Design review of the part built by this model. Coordinates are the model's own, in mm. Face numbers are marked on the shaded views. A direction names the side the tool comes from. Coordinates: 2 decimals unless noted, no trailing zeros. Write each loop counter-clockwise with the first axis right and the second up, starting at its lowest first coordinate (ties: lowest second). Pieces come first, ordered by that corner, then holes. Notation, with made-up numbers: (16, 42) -> (34, 42) arc R21 ccw to (34, 80) -> close; hole circle Ø6 at (62, 50.5). An arc over 180 degrees is marked (long way). Write item = value, one per line. Start each with the question number.
```python
from build123d import *


with BuildPart() as part:
    # Sketch1 → Revolve1 (revolve)
    with BuildSketch(Plane(origin=(0, 0, 0), x_dir=(1, 0, 0), z_dir=(0, 1, 0)), mode=Mode.PRIVATE) as revolve1_sk:
        with BuildLine():
            Line((-7.95, 11.1), (-0.95, 11.1))
            Line((-0.95, 11.1), (-0.95, 6.1))
            Line((-0.95, 6.1), (0.95, 6.1))
            Line((0.95, 6.1), (0.95, 11.1))
            Line((0.95, 11.1), (7.95, 11.1))
            Line((7.95, 11.1), (7.95, 21))
            Line((7.95, 21), (6.75, 21))
            Line((6.75, 21), (3.703703704, 17.641044973))
            ThreePointArc((3.703703704, 17.641044973), (0, 16), (-3.703703704, 17.641044973))
            Line((-3.703703704, 17.641044973), (-6.75, 21))
            Line((-6.75, 21), (-7.95, 21))
            Line((-7.95, 21), (-7.95, 11.1))
        make_face()
    revolve(revolve1_sk.sketch.rotate(Axis((-3.715814159, 0, 0), (1, 0, 0)), 180), axis=Axis((-3.715814159, 0, 0), (1, 0, 0)))


solid = part.part
```
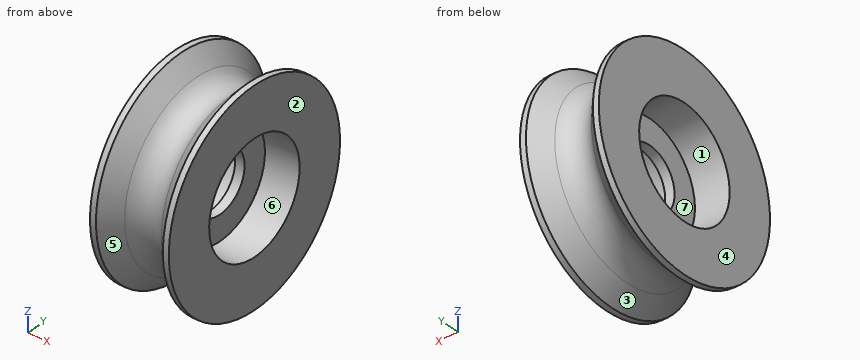
(1) Take a section at A-A, the plane y = 0. State the section outline as (x, z) points.
(2) For pin 1 Ø18 at (y, z) = (0, 0) entering from +X; pin 2 Ø3 at (x, y) = (-3, -15.5) entering from -Z; pin 3 Ø3 at (x, y) = (5.5, 5.5) entering from -Z, all flat-tipped, find the tip position at first contact; note any pin that passes through.
(3) For the marked faces 4, 5, 6 and 7, list the 3-axis set-ups (+Z, -Z, +X, -X, +Y, -Y) from which the entire face can be reached by the end or side of a thin tool; tool diameter is ignored.
(4) For line 1 (Y direction, x = -5, z = -1); line 2 (Y direction, x = -5.5, z = -8.5); line 3 (Z direction, x = -6.5, y = -5.5), list the stretches that pass through material, from the lowest coordinate up.
(5) Take a section at C-C, the plane x = 6. State the section outline as (y, z) points, then the cut area to 3 significant figures.
(6) Take a section at D-D, the plane x = 2.75. State the section outline as (y, z) points.
(7) Mouldability with a two-part tool opening along X and no side actions: class the marked faces 1, 2 and 3 as pulls with the +X half, pulls with the -X half, needs draft (parallel to the pull), parting line crosses it, or undercut.
Report:
q1.outline = (-7.95, -21) -> (-6.75, -21) -> (-3.7, -17.64) arc R5 cw to (3.7, -17.64) -> (6.75, -21) -> (7.95, -21) -> (7.95, -11.1) -> (0.95, -11.1) -> (0.95, -6.1) -> (-0.95, -6.1) -> (-0.95, -11.1) -> (-7.95, -11.1) -> close; (-7.95, 11.1) -> (-0.95, 11.1) -> (-0.95, 6.1) -> (0.95, 6.1) -> (0.95, 11.1) -> (7.95, 11.1) -> (7.95, 21) -> (6.75, 21) -> (3.7, 17.64) arc R5 cw to (-3.7, 17.64) -> (-6.75, 21) -> (-7.95, 21) -> close
q2.pin_1 = 0.95
q2.pin_2 = -10.85
q2.pin_3 = -20.47
q3.face_4 = +Z, -Z, -X, +Y, -Y
q3.face_5 = none
q3.face_6 = +X
q3.face_7 = -X
q4.line_1 = -19.04 to -11.05, 11.05 to 19.04
q4.line_2 = -17.69 to -7.14, 7.14 to 17.69
q4.line_3 = -19.98 to -9.64, 9.64 to 19.98
q5.outline = circle Ø40.35 at (0, 0); hole circle Ø22.2 at (0, 0)
q5.area = 891 mm2
q6.outline = circle Ø33.65 at (0, 0); hole circle Ø22.2 at (0, 0)
q7.face_1 = needs draft
q7.face_2 = pulls with the +X half
q7.face_3 = undercut
